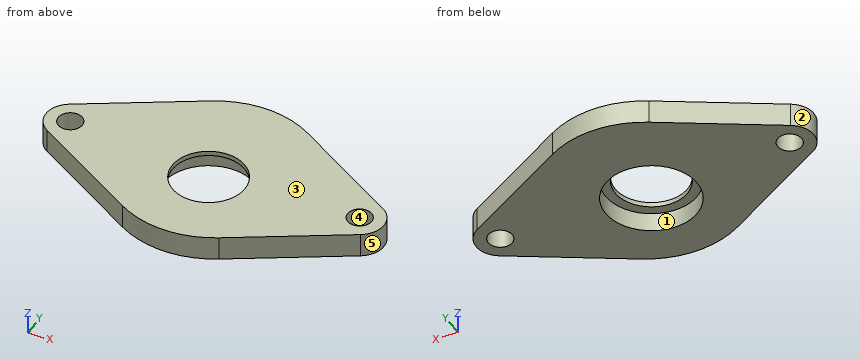
from build123d import *

# Parameters (mm, degrees)
BOSS_EXTRUDE1_DEPTH = 10
SKETCH1_3_R         = 15
SKETCH1_3_R_2       = 5
CUT_EXTRUDE1_DEPTH  = 10
SKETCH1_4_R         = 19
CUT_EXTRUDE2_DEPTH  = 8


with BuildPart() as part:
    # Sketch1 → Boss-Extrude1 (new body)
    with BuildSketch(Plane.XY):
        with BuildLine():
            Line((-20, 99.641016151), (-65, 73.660254038))
            ThreePointArc((-65, 73.660254038), (-70, 65), (-65, 56.339745962))
            Line((-65, 56.339745962), (-20, 30.358983849))
            ThreePointArc((-20, 30.358983849), (0, 25), (20, 30.358983849))
            Line((20, 30.358983849), (65, 56.339745962))
            ThreePointArc((65, 56.339745962), (70, 65), (65, 73.660254038))
            Line((65, 73.660254038), (20, 99.641016151))
            ThreePointArc((20, 99.641016151), (0, 105), (-20, 99.641016151))
        make_face()
    extrude(amount=BOSS_EXTRUDE1_DEPTH)

    # Sketch1<3> → Cut-Extrude1 (cut)
    with BuildSketch(Plane.XY):
        with Locations((0, 60)):
            Circle(SKETCH1_3_R)
        with Locations((-60, 65)):
            Circle(SKETCH1_3_R_2)
        with Locations((60, 65)):
            Circle(SKETCH1_3_R_2)
    extrude(amount=CUT_EXTRUDE1_DEPTH, mode=Mode.SUBTRACT)

    # Sketch1<4> → Cut-Extrude2 (cut)
    with BuildSketch(Plane.XY):
        with Locations((0, 60)):
            Circle(SKETCH1_4_R)
    extrude(amount=CUT_EXTRUDE2_DEPTH, mode=Mode.SUBTRACT)


solid = part.part
Check sheet for the modelled part. Datum: model origin and axes. Units: mm. Face numbers are marked on the shaded views. A direction names the side the tool comes from. Give positions to 0.01 mm unless a question says otherwise; leave off trailing zeros. Write each loop counter-clockwise with the first axis right and the second up, starting at its lowest first coordinate (ties: lowest second). Pieces come first, ordered by that corner, then holes. Notation, with made-up numbers: (46.25, 64) -> (75.25, 64) arc R28 ccw to (75.25, 94) -> close; hole circle Ø2 at (25.5, -38.75). An arc over 180 degrees is marked (long way). Write item = value, one per line.
Item 1: Sectioned sample at B-B on x = 0. Record the boundary of the cut face in (y, z), and give its area (3 significant figures).
Output:
outline = (25, 0) -> (41, 0) -> (41, 8) -> (45, 8) -> (45, 10) -> (25, 10) -> close; (75, 8) -> (79, 8) -> (79, 0) -> (105, 0) -> (105, 10) -> (75, 10) -> close
area = 436 mm^2
Item 2: Tool access check on the marked faces 1 and 2. Record the directions out of +Z, -Z, +X, -X, +Y, -Y that give a thin tool (end or side, any length) a straight path to the whole face; none if there is none.
Output:
face_1 = -Z
face_2 = +Z, -Z, -X
Item 3: Gauge pin test, flat ends, axial feed: pin 1 (13 mm diameter, centred on x = 60, y = 65, fed in from -Z); pin 2 (24 mm diameter, centred on x = 0, y = 60, fed in from +Z); pin 3 (2 mm diameter, centred on x = 52.5, z = 6, fed in from -Y); pin 4 (2 mm diameter, centred on y = 58.5, z = 7.5, fed in from +X). Record the tip position at first contact, or that the pin passes through.
Output:
pin_1 = 0
pin_2 = through
pin_3 = 48.55
pin_4 = 68.35
Item 4: Scan lines: probe 1 along X at (y, z) = (60.5, 4.5); probe 2 along Z at (x, y) = (-1.5, 44.5); probe 3 along Y at (x, z) = (-5.5, 3). Record each from-to range of solid material in increasing order. Write a range as from..to.
Output:
probe_1 = -68.93..-62.18, -57.82..-18.99, 18.99..57.82, 62.18..68.93
probe_2 = 8..10
probe_3 = 25.38..41.81, 78.19..104.62
Item 5: Release check for a two-part mould opening along X. For the marked faces 3, 4 and 5 record: +X half, -X half, draft (parallel to the pull), parting line (faces both ways), or undercut.
Output:
face_3 = draft
face_4 = undercut
face_5 = +X half
Item 6: Sectioned sample at C-C on y = 67.5. Record the boundary of the cut face in (x, z), and give its area (3 significant figures).
Output:
outline = (-69.68, 0) -> (-64.33, 0) -> (-64.33, 10) -> (-69.68, 10) -> close; (-55.67, 0) -> (-17.46, 0) -> (-17.46, 8) -> (-12.99, 8) -> (-12.99, 10) -> (-55.67, 10) -> close; (12.99, 8) -> (17.46, 8) -> (17.46, 0) -> (55.67, 0) -> (55.67, 10) -> (12.99, 10) -> close; (64.33, 0) -> (69.68, 0) -> (69.68, 10) -> (64.33, 10) -> close
area = 889 mm^2
Item 7: Sectioned sample at D-D on x = 60. Record the boundary of the cut face in (y, z).
Output:
outline = (53.45, 0) -> (60, 0) -> (60, 10) -> (53.45, 10) -> close; (70, 0) -> (76.55, 0) -> (76.55, 10) -> (70, 10) -> close
Item 8: Sectioned sample at A-A on z = 2.5. Record the boundary of the cut face in (x, y).
Output:
outline = (-65, 56.34) -> (-20, 30.36) arc R40 ccw to (20, 30.36) -> (65, 56.34) arc R10 ccw to (65, 73.66) -> (20, 99.64) arc R40 ccw to (-20, 99.64) -> (-65, 73.66) arc R10 ccw to start; hole circle Ø10 at (-60, 65); hole circle Ø38 at (0, 60); hole circle Ø10 at (60, 65)
